from build123d import *

# Parameters (mm, degrees)
F0_W     = 12.7
F0_H     = 25.4
F0_H_2   = 12.7
F1_DEPTH = 6.35


with BuildPart() as f1:
    # F0 (on Top) → F1 (new body)
    with BuildSketch(Plane.XY):
        with Locations((6.35, 12.7)):
            Rectangle(F0_W, F0_H)
        with Locations((-6.35, 31.75)):
            Rectangle(F0_W, F0_H_2)
        with Locations((6.35, 31.75)):
            Rectangle(F0_W, F0_H_2)
        with Locations((19.05, 31.75)):
            Rectangle(F0_W, F0_H_2)
        with Locations((6.35, 44.45)):
            Rectangle(F0_W, F0_H_2)
    extrude(amount=F1_DEPTH)


solid = f1.part
Could you check a few things on this model? Use its own coordinates, in mm. A direction names the side the tool comes from. Coordinates: 2 decimals unless noted, no trailing zeros. Loops run counter-clockwise (first coordinate to the right, second up) from the corner with the lowest first, then second, coordinate; pieces in that order, holes last.
1. I need wall thicknesses on L1, parallel to X at y = 12.5, z = 6; L2, parallel to Y at x = -8, z = 0.5. Which ranges of each line are inside material? Lowest first, please.
2. Imagine slicing it at C-C (x = -8.5). Please give me the cut outline in (y, z).
3. For P1, Ø4, axis at x = 12, y = 13, coming from the -Z side; P2, Ø3, axis at y = 18, z = 1.5, coming from the +X side; P3, Ø1.5, axis at x = -8, z = 3, coming from the +Y side; P4, Ø1.9, axis at y = 46, z = 4.5, coming from the -X side, each with a flat end and sliding along its axis, tell me the tip position at first contact or that it passes through.
4. Imagine slicing it at A-A (z = 2.75). Please give me the cut outline in (x, y), and give its area (3 significant figures).
5. For faces 1 (the face through (0, 13, 3)), 2 (the face through (-6, 38.1, 3)), 3 (the face through (25.4, 32, 3)), 4 (the face through (19, 38.1, 3)), 5 (the face through (19, 25.4, 3)), which set-ups out of +Z, -Z, +X, -X, +Y, -Y let a thin tool reach every point of the face, with its end or its side?
6. Imagine slicing it at B-B (y = 9.5). Please give me the cut outline in (x, z).
Computed values:
1. L1: x = 0 to 12.7
1. L2: y = 25.4 to 38.1
2. outline: (25.4, 0) - (38.1, 0) - (38.1, 6.35) - (25.4, 6.35) - close
3. P1: stops at z = 0
3. P2: stops at x = 12.7
3. P3: stops at y = 38.1
3. P4: stops at x = 0
4. outline: (-12.7, 25.4) - (0, 25.4) - (0, 0) - (12.7, 0) - (12.7, 25.4) - (25.4, 25.4) - (25.4, 38.1) - (12.7, 38.1) - (12.7, 50.8) - (0, 50.8) - (0, 38.1) - (-12.7, 38.1) - close
4. area: 968 mm2
5. face 1: +Z, -Z, -X, -Y
5. face 2: +Z, -Z, -X, +Y
5. face 3: +Z, -Z, +X, +Y, -Y
5. face 4: +Z, -Z, +X, +Y
5. face 5: +Z, -Z, +X, -Y
6. outline: (0, 0) - (12.7, 0) - (12.7, 6.35) - (0, 6.35) - close
